```python
from build123d import *

# Parameters (mm, degrees)
SKETCH1_W           = 22.5
SKETCH1_H           = 9.6
BOSS_EXTRUDE1_DEPTH = 11.5
CUT_EXTRUDE1_DEPTH  = 19.73426006
SKETCH4_W           = 8.75
SKETCH4_H           = 7.8
CUT_EXTRUDE2_DEPTH  = 2.6
SKETCH5_R           = 1.325
CUT_EXTRUDE3_DEPTH  = 17.119941067
CHAMFER1_SIZE       = 0.75
SKETCH6_W           = 3.6
SKETCH6_H           = 1.175
CUT_EXTRUDE4_DEPTH  = 2.4


with BuildPart() as part:
    # Sketch1 → Boss-Extrude1 (new body)
    with BuildSketch(Plane(origin=(0, 0, 0), x_dir=(1, 0, 0), z_dir=(0, 1, 0))):
        Rectangle(SKETCH1_W, SKETCH1_H)
    extrude(amount=BOSS_EXTRUDE1_DEPTH)

    # Sketch3 → Cut-Extrude1 (cut, through all)
    with BuildSketch(Plane.XY.offset(4.8)):
        Polygon((4.75, 11.5), (4.375, 3.6), (-4.375, 3.6), (-4.75, 11.5), align=None)
    extrude(amount=-CUT_EXTRUDE1_DEPTH, mode=Mode.SUBTRACT)

    # Sketch4 → Cut-Extrude2 (cut)
    with BuildSketch(Plane(origin=(0, 3.6, 0), x_dir=(1, 0, 0), z_dir=(0, 1, 0))):
        Rectangle(SKETCH4_W, SKETCH4_H)
    extrude(amount=-CUT_EXTRUDE2_DEPTH, mode=Mode.SUBTRACT)

    # Sketch5 → Cut-Extrude3 (cut, through all)
    with BuildSketch(Plane(origin=(0, 1, 0), x_dir=(1, 0, 0), z_dir=(0, 1, 0))):
        with Locations(Location((0, 0, 0), (0, 0, 270))):
            Circle(SKETCH5_R)
    extrude(amount=-CUT_EXTRUDE3_DEPTH, mode=Mode.SUBTRACT)

    # Chamfer1
    chamfer1_edges = [part.edges().sort_by_distance(p)[0] for p in [
        (0, 1, -1.325),
    ]]
    chamfer(chamfer1_edges, length=CHAMFER1_SIZE)

    # Sketch6 → Cut-Extrude4 (cut)
    with BuildSketch(Plane.XZ):
        with Locations((0, 4.2125)):
            Rectangle(SKETCH6_W, SKETCH6_H)
    cut_extrude4 = extrude(amount=-CUT_EXTRUDE4_DEPTH, mode=Mode.SUBTRACT)

    # Mirror1: Cut-Extrude4 across plane
    add(cut_extrude4.mirror(Plane.XY), mode=Mode.SUBTRACT)


solid = part.part
```
CAD build for the part. Positions are in the model's coordinates, mm. A direction names the side the tool comes from. Round coordinates to 2 decimals unless told otherwise and drop trailing zeros. Order: outer loops, then holes, each group sorted by start corner. A loop starts at its lowest first (then second) coordinate and runs counter-clockwise, first axis right, second up. Notation, with made-up numbers: (38.5, 31.5) -> (51.5, 31.5) arc R23 ccw to (51.5, 60.5) -> close; hole circle Ø9 at (65.5, -11.5). An arc over 180 degrees is marked (long way). One line per question, with ' | ' between items.
Q1. Slice it at C-C (x = 0). Write the cut outline in (y, z) (3 decimals).
Completed:
outline: (0, -3.625) -> (1, -3.625) -> (1, -2.075) -> (0.25, -1.325) -> (0, -1.325) -> close; (0, 1.325) -> (0.25, 1.325) -> (1, 2.075) -> (1, 3.625) -> (0, 3.625) -> close; (2.4, -4.8) -> (3.6, -4.8) -> (3.6, -3.9) -> (2.4, -3.9) -> close; (2.4, 3.9) -> (3.6, 3.9) -> (3.6, 4.8) -> (2.4, 4.8) -> close
Q2. Which spindle directions (+Z, -Z, +X, -X, +Y, -Y) get a long thin tool onto all of the face, cutting with end or side? Do faces 1 (the flat face through (1.8, 1.2, 4.2)), 2 (the flat face through (0, 0.5, 3.625)), 3 (the flat face through (-4.375, 2, 0)), 4 (the flat face through (-4.56, 7.49, 0.07)). Say none if no direction does.
Completed:
face 1: +Z, -Y | face 2: +Z, +Y, -Y | face 3: +Y | face 4: +Z, -Z, +Y
Q3. Slice it at D-D (x = 3.5). Write the cut outline in (y, z), then the cut area to 3 significant figures.
Completed:
outline: (0, -4.8) -> (3.6, -4.8) -> (3.6, -3.9) -> (1, -3.9) -> (1, 3.9) -> (3.6, 3.9) -> (3.6, 4.8) -> (0, 4.8) -> close | area: 14.3 mm^2
Q4. Drop flat-ended pins along their axis: pin 1 (0.5 mm diameter, centred on x = -0.5, z = -4.5, fed in from -Y); pin 2 (0.7 mm diameter, centred on x = -1.5, z = 4, fed in from +Y); pin 3 (1.1 mm diameter, centred on x = -0.5, y = 0.5, fed in from +Z) (3 decimals). Give the stop position or say it passes through.
Completed:
pin 1: stops at y = 2.4 | pin 2: stops at y = 3.6 | pin 3: stops at z = 3.625
Q5. Slice it at A-A (z = 0). Write the cut outline in (x, y) (3 decimals).
Completed:
outline: (-11.25, 0) -> (-1.325, 0) -> (-1.325, 0.25) -> (-2.075, 1) -> (-4.375, 1) -> (-4.375, 3.6) -> (-4.75, 11.5) -> (-11.25, 11.5) -> close; (1.325, 0) -> (11.25, 0) -> (11.25, 11.5) -> (4.75, 11.5) -> (4.375, 3.6) -> (4.375, 1) -> (2.075, 1) -> (1.325, 0.25) -> close
Q6. Probe probe 1 along X at (y, z) = (0.1, 0) (3 decimals); probe 2 along Z at (x, y) = (-3, 2); probe 3 along X at (y, z) = (2.75, 1.75) (3 decimals). List the from-to ranges inside material, lowest first.
Completed:
probe 1: x = -11.25 to -1.325, 1.325 to 11.25 | probe 2: z = -4.8 to -3.9, 3.9 to 4.8 | probe 3: x = -11.25 to -4.375, 4.375 to 11.25
Q7. Two-plate mould, pull along Z, no slides. Class faces 5 (the flat face through (0.1, 3.6, 4.4)), 6 (the flat face through (0, 0.5, -3.625)), 7 (the flat face through (4.375, 2, 0)), 8 (the flat face through (0, 3, 4.8)): released by +Z, released by -Z, zero draft, split by the parting line, or undercut.
Completed:
face 5: zero draft | face 6: released by -Z | face 7: undercut | face 8: released by +Z
Q8. Slice it at B-B (y = 1.5). Write the cut outline in (x, z) (3 decimals).
Completed:
outline: (-11.25, -4.8) -> (-1.8, -4.8) -> (-1.8, -3.9) -> (-4.375, -3.9) -> (-4.375, 3.9) -> (-1.8, 3.9) -> (-1.8, 4.8) -> (-11.25, 4.8) -> close; (1.8, -4.8) -> (11.25, -4.8) -> (11.25, 4.8) -> (1.8, 4.8) -> (1.8, 3.9) -> (4.375, 3.9) -> (4.375, -3.9) -> (1.8, -3.9) -> close
